```python
from build123d import *

# Parameters (mm, degrees)
SKETCH1_W                  = 20
SKETCH1_H                  = 242.6825
SKETCH1_R                  = 2.35
BASE_FLANGE1_DEPTH         = 1.016
SKETCHED_START             = -20
SKETCHED_BEND1_DEPTH       = 20
SKETCHED_BEND1_2_DEPTH     = 7.6499999
SKETCHED_START_2           = -7.6499999
SKETCHED_BEND1_3_DEPTH     = 7.6499999
SKETCHED_START_3           = -12.3500001
SKETCHED_BEND1_4_DEPTH     = 4.7000002
SKETCHED_START_4           = 58.325262761
SKETCHED_BEND1_5_OUTLINE_R = 2.35
SKETCHED_BEND1_5_DEPTH     = 126.031974478
SKETCH7_R                  = 2.35
CUT_EXTRUDE1_DEPTH         = 10
SKETCH8_W                  = 14
SKETCH8_H                  = 4
CUT_EXTRUDE2_DEPTH         = 1.016


with BuildPart() as part:
    # Base-Flange1: sheet metal written as solids
    # Sketch1 → Base-Flange1 (new body)
    with BuildSketch(Plane.XY):
        with Locations((-10, 121.34125)):
            Rectangle(SKETCH1_W, SKETCH1_H)
        with Locations((-10, 28.5)):
            Circle(SKETCH1_R, mode=Mode.SUBTRACT)
        with Locations((-10, 10.5)):
            Circle(SKETCH1_R, mode=Mode.SUBTRACT)
        with Locations((-10, 232.1825)):
            Circle(SKETCH1_R, mode=Mode.SUBTRACT)
        with Locations((-10, 214.1825)):
            Circle(SKETCH1_R, mode=Mode.SUBTRACT)
    extrude(amount=-BASE_FLANGE1_DEPTH)

    # Sketched Bend1: read off the stored shape, not the designer's step
    # Sketched Bend1 outline → Sketched Bend1 (cut)
    with BuildSketch(Plane.YZ.offset(SKETCHED_START)):
        with BuildLine():
            ThreePointArc((184.238608772, 0), (183.640375265, -0.738276315), (182.731637239, -1.016))
            Line((182.731637239, -1.016), (242.6825, -1.016))
            Line((242.6825, -1.016), (242.6825, 0))
            Line((242.6825, 0), (184.238608772, 0))
        make_face()
        with BuildLine():
            Line((0, -1.016), (59.950862761, -1.016))
            ThreePointArc((59.950862761, -1.016), (59.042124735, -0.738276315), (58.443891228, 0))
            Line((58.443891228, 0), (0, 0))
            Line((0, 0), (0, -1.016))
        make_face()
    extrude(amount=SKETCHED_BEND1_DEPTH, mode=Mode.SUBTRACT)

    # Sketched Bend1 2 outline → Sketched Bend1 2 (add)
    with BuildSketch(Plane.YZ.offset(SKETCHED_START)):
        with BuildLine():
            Line((182.731637239, 0), (184.238608772, 0))
            ThreePointArc((184.238608772, 0), (184.327304542, 0.299082338), (184.357237239, 0.6096))
            Line((184.357237239, 0.6096), (184.357237239, 58.884737239))
            Line((184.357237239, 58.884737239), (183.341237239, 58.884737239))
            Line((183.341237239, 58.884737239), (183.341237239, 0.6096))
            ThreePointArc((183.341237239, 0.6096), (183.162689533, 0.178547706), (182.731637239, 0))
        make_face()
        with BuildLine():
            ThreePointArc((58.325262761, 0.6096), (58.355195458, 0.299082338), (58.443891228, 0))
            Line((58.443891228, 0), (59.950862761, 0))
            ThreePointArc((59.950862761, 0), (59.519810467, 0.178547706), (59.341262761, 0.6096))
            Line((59.341262761, 0.6096), (59.341262761, 58.884737239))
            Line((59.341262761, 58.884737239), (58.325262761, 58.884737239))
            Line((58.325262761, 58.884737239), (58.325262761, 0.6096))
        make_face()
    extrude(amount=SKETCHED_BEND1_2_DEPTH)

    # Sketched Bend1 3 outline → Sketched Bend1 3 (add)
    with BuildSketch(Plane.YZ.offset(SKETCHED_START_2)):
        with BuildLine():
            Line((182.731637239, 0), (184.238608772, 0))
            ThreePointArc((184.238608772, 0), (184.327304542, 0.299082338), (184.357237239, 0.6096))
            Line((184.357237239, 0.6096), (184.357237239, 58.884737239))
            Line((184.357237239, 58.884737239), (183.341237239, 58.884737239))
            Line((183.341237239, 58.884737239), (183.341237239, 0.6096))
            ThreePointArc((183.341237239, 0.6096), (183.162689533, 0.178547706), (182.731637239, 0))
        make_face()
        with BuildLine():
            ThreePointArc((58.325262761, 0.6096), (58.355195458, 0.299082338), (58.443891228, 0))
            Line((58.443891228, 0), (59.950862761, 0))
            ThreePointArc((59.950862761, 0), (59.519810467, 0.178547706), (59.341262761, 0.6096))
            Line((59.341262761, 0.6096), (59.341262761, 58.884737239))
            Line((59.341262761, 58.884737239), (58.325262761, 58.884737239))
            Line((58.325262761, 58.884737239), (58.325262761, 0.6096))
        make_face()
    extrude(amount=SKETCHED_BEND1_3_DEPTH)

    # Sketched Bend1 4 outline → Sketched Bend1 4 (add)
    with BuildSketch(Plane.YZ.offset(SKETCHED_START_3)):
        with BuildLine():
            Line((182.731637239, 0), (184.238608772, 0))
            ThreePointArc((184.238608772, 0), (184.327304542, 0.299082338), (184.357237239, 0.6096))
            Line((184.357237239, 0.6096), (184.357237239, 58.884737239))
            Line((184.357237239, 58.884737239), (183.341237239, 58.884737239))
            Line((183.341237239, 58.884737239), (183.341237239, 0.6096))
            ThreePointArc((183.341237239, 0.6096), (183.162689533, 0.178547706), (182.731637239, 0))
        make_face()
        with BuildLine():
            Line((58.443891228, 0), (59.950862761, 0))
            ThreePointArc((59.950862761, 0), (59.519810467, 0.178547706), (59.341262761, 0.6096))
            Line((59.341262761, 0.6096), (59.341262761, 58.884737239))
            Line((59.341262761, 58.884737239), (58.325262761, 58.884737239))
            Line((58.325262761, 58.884737239), (58.325262761, 0.6096))
            ThreePointArc((58.325262761, 0.6096), (58.355195458, 0.299082338), (58.443891228, 0))
        make_face()
    extrude(amount=SKETCHED_BEND1_4_DEPTH)

    # Sketched Bend1 5 outline → Sketched Bend1 5 (cut)
    with BuildSketch(Plane(origin=(0, 0, 0), x_dir=(1, 0, 0), z_dir=(0, 1, 0)).offset(SKETCHED_START_4)):
        with Locations((-10, -30.384737239)):
            Circle(SKETCHED_BEND1_5_OUTLINE_R)
        with Locations((-10, -48.384737239)):
            Circle(SKETCHED_BEND1_5_OUTLINE_R)
    extrude(amount=SKETCHED_BEND1_5_DEPTH, mode=Mode.SUBTRACT)

    # Sketch7 → Cut-Extrude1 (cut)
    with BuildSketch(Plane(origin=(0, 0, -1.016), x_dir=(-1, 0, 0), z_dir=(0, 0, -1))):
        with Locations((9.918784011, 73.325262761)):
            Circle(SKETCH7_R)
        with Locations((10, 169.357237239)):
            Circle(SKETCH7_R)
    extrude(amount=-CUT_EXTRUDE1_DEPTH, mode=Mode.SUBTRACT)

    # Sketch8 → Cut-Extrude2 (cut)
    with BuildSketch(Plane(origin=(0, 0, -1.016), x_dir=(-1, 0, 0), z_dir=(0, 0, -1))):
        with Locations((10, 149.34125)):
            Rectangle(SKETCH8_W, SKETCH8_H)
        with Locations((10, 142.34125)):
            Rectangle(SKETCH8_W, SKETCH8_H)
        with Locations((10, 135.34125)):
            Rectangle(SKETCH8_W, SKETCH8_H)
        with Locations((10, 128.34125)):
            Rectangle(SKETCH8_W, SKETCH8_H)
        with Locations((10, 121.34125)):
            Rectangle(SKETCH8_W, SKETCH8_H)
        with Locations((10, 114.34125)):
            Rectangle(SKETCH8_W, SKETCH8_H)
        with Locations((10, 107.34125)):
            Rectangle(SKETCH8_W, SKETCH8_H)
        with Locations((10, 100.34125)):
            Rectangle(SKETCH8_W, SKETCH8_H)
        with Locations((10, 93.34125)):
            Rectangle(SKETCH8_W, SKETCH8_H)
    extrude(amount=-CUT_EXTRUDE2_DEPTH, mode=Mode.SUBTRACT)


solid = part.part
```
Here's how the part is built. I have some questions about the finished solid (model axes, mm). A direction names the side the tool comes from. Round coordinates to 2 decimals unless told otherwise and drop trailing zeros. Order: outer loops, then holes, each group sorted by start corner. A loop starts at its lowest first (then second) coordinate and runs counter-clockwise, first axis right, second up. Notation, with made-up numbers: M 10,-2.75 L 63,-2.75 A25 ccw 63,9.25 Z; hole C 35,1.5 d10. An arc over 180 degrees is marked long. One line per question, with ' | ' between items.
1) For pin 1 Ø0.8 at (x, z) = (-9.5, -0.5) entering from -Y; pin 2 Ø0.5 at (y, z) = (108, -0.5) entering from +X; pin 3 Ø1.5 at (x, y) = (-6.5, 74.5) entering from +Z; pin 4 Ø0.5 at (x, z) = (-12.5, -0.5) entering from +Y, each with a flat end and sliding along its axis, tell me the tip position at first contact or that it passes through.
Working result:
pin 1: y = 58.49 | pin 2: x = 0 | pin 3: z = 0 | pin 4: y = 184.11
2) For faces 4 (the face through (-15, 183.341, 30)), 5 (the face through (-15, 58.325, 30)), which set-ups out of +Z, -Z, +X, -X, +Y, -Y let a thin tool reach every point of the face, with its end or its side?
Working result:
face 4: +Z, +X, -X | face 5: +Z, -Z, +X, -X, -Y
3) If we mould it in two halves opening along X, with no side actions, what happens to faces 1 (the face through (-12.4, 59.341, 29.3)), 2 (the face through (-12.348, 183.842, 30.281)), 3 (the face through (-9.613, 75.655, -0.515))? For each: +X half, -X half, draft (parallel to the pull), parting line (faces both ways), or undercut.
Working result:
face 1: draft | face 2: undercut | face 3: undercut
4) I want a section at C-C, the plane x = -1.5. Write out the boundary of the cut face in (y, z), then the cut area to 3 significant figures.
Working result:
outline: M 58.33,0.61 A1.63 ccw 59.95,-1.02 L 182.73,-1.02 A1.63 ccw 184.36,0.61 L 184.36,58.88 L 183.34,58.88 L 183.34,0.61 A0.61 cw 182.73,0 L 59.95,0 A0.61 cw 59.34,0.61 L 59.34,58.88 L 58.33,58.88 Z | area: 247 mm²
5) I want a section at A-A, the plane y = 142.5. Write out the boundary of the cut face in (x, z), then the cut area to 3 significant figures.
Working result:
outline: M -20,-1.02 L -17,-1.02 L -17,0 L -20,0 Z; M -3,-1.02 L 0,-1.02 L 0,0 L -3,0 Z | area: 6.10 mm²
6) I need wall thicknesses on line 1 along Y through (x, z) = (-8.5, 44); line 2 along Z through (x, y) = (-7, 97); line 3 along Z through (x, y) = (-10, 58.7). Which ranges of each line are inside material? Lowest first, please.
Working result:
line 1: 58.33 to 59.34, 183.34 to 184.36 | line 2: -1.02 to 0 | line 3: -0.43 to 28.03, 32.73 to 46.03, 50.73 to 58.88
7) I want a section at D-D, the plane x = -10. State how many separate pieces and enclosed holes the cut face has, then the cut area to 3 significant figures.
Working result:
separate pieces: 16 | enclosed holes: 0 | area: 182 mm²
8) I want a section at B-B, the plane z = 52.5. Write out the boundary of the cut face in (x, y).
Working result:
outline: M -20,58.33 L 0,58.33 L 0,59.34 L -20,59.34 Z; M -20,183.34 L 0,183.34 L 0,184.36 L -20,184.36 Z
